```python
from build123d import *

# Parameters (mm, degrees)
EXTRUDE_366_DEPTH           = 3.75
EXTRUDE_366_TAPER           = 4.000000000000009
EXTRUDE_366_OTHER_WAY_DEPTH = 3.75
EXTRUDE_366_OTHER_WAY_TAPER = 4.000000000000009
EXTRUDE_746_DEPTH           = 3.75
EXTRUDE_746_TAPER           = 4.000000000000009
CUT_EXTRUDE_1239_DEPTH      = 10
SKETCH_4_R                  = 10
CUT_EXTRUDE_1_DEPTH         = 10
EXTRUDE_1783_DEPTH          = 7
FILLET_2_R                  = 2
FILLET_3_R                  = 2


with BuildPart() as part:
    # Эскиз1 → Extrude 366 (new body)
    with BuildSketch(Plane.XY):
        with BuildLine():
            ThreePointArc((-0.9374999999999997, 14.970674458754353), (-15.000000000000044, 1.84e-15), (-0.9374999999999997, -14.970674458754353))
            Line((-0.9374999999999997, -14.970674458754353), (78.75, -19.960899278339134))
            ThreePointArc((78.75, -19.960899278339134), (100, 0), (78.75, 19.960899278339134))
            Line((78.75, 19.960899278339134), (-0.9374999999999997, 14.970674458754353))
        make_face()
    extrude(amount=EXTRUDE_366_DEPTH, taper=EXTRUDE_366_TAPER)

    # Эскиз1 → Extrude 366 other way (add)
    with BuildSketch(Plane.XY):
        with BuildLine():
            ThreePointArc((-0.9374999999999997, 14.970674458754353), (-15.000000000000044, 1.84e-15), (-0.9374999999999997, -14.970674458754353))
            Line((-0.9374999999999997, -14.970674458754353), (78.75, -19.960899278339134))
            ThreePointArc((78.75, -19.960899278339134), (100, 0), (78.75, 19.960899278339134))
            Line((78.75, 19.960899278339134), (-0.9374999999999997, 14.970674458754353))
        make_face()
    extrude(amount=-EXTRUDE_366_OTHER_WAY_DEPTH, taper=EXTRUDE_366_OTHER_WAY_TAPER)

    # Эскиз2 → Extrude 746 (add)
    with BuildSketch(Plane.XY):
        with BuildLine():
            Line((-8.829475928589163, 70.3052843721409), (28.552506867722524, 0))
            Line((28.552506867722524, 0), (62.650318248221396, 1.896e-14))
            Line((62.650318248221396, 1.896e-14), (8.2903757255504, 80.59192903470749))
            ThreePointArc((8.2903757255504, 80.59192903470749), (-5.150380749100648, 83.57167300702106), (-8.829475928589163, 70.3052843721409))
        make_face()
    extrude(amount=EXTRUDE_746_DEPTH, taper=EXTRUDE_746_TAPER)

    # Эскиз3 → Cut-Extrude 1239 (cut)
    with BuildSketch(Plane.XY.offset(3.75)):
        with BuildLine():
            Line((3.464101615137748, 77.00000000000001), (23.464101615137906, 42.35898384862258))
            ThreePointArc((23.464101615137906, 42.35898384862258), (22.00000000000019, 36.89488223348481), (16.53589838486241, 38.358983848622536))
            Line((16.53589838486241, 38.358983848622536), (-3.464101615137746, 72.99999999999997))
            ThreePointArc((-3.464101615137746, 72.99999999999997), (-2.00000000000002, 78.46410161513775), (3.464101615137748, 77.00000000000001))
        make_face()
    extrude(amount=-CUT_EXTRUDE_1239_DEPTH, mode=Mode.SUBTRACT)

    # Эскиз4 → отверстие1 (cut)
    with BuildSketch(Plane.XY.offset(3.75)):
        Circle(SKETCH_4_R)
    extrude(amount=-CUT_EXTRUDE_1_DEPTH, mode=Mode.SUBTRACT)

    # Эскиз5 → Extrude 1783 (add)
    with BuildSketch(Plane.XY.offset(3.75)):
        Polygon((79.99999999999999, 13.856406460551018), (68, 6.928203230275526), (68, -6.9282032302754955), (80, -13.856406460551012), (92, -6.928203230275516), (92, 6.928203230275502), align=None)
    extrude(amount=EXTRUDE_1783_DEPTH)

    # Скругление2
    fillet_2_edges = [part.edges().sort_by_distance(p)[0] for p in [
        (99.73777445521183, -1.332e-14, -3.75),
        (99.73777445521183, -3.77e-15, 3.7499999999999996),
        (9.700092064405581, 15.374087104269854, 3.7499999999999987),
        (-14.737774455211877, -5.44e-15, 3.7499999999999996),
        (38.922639096549254, -17.204073984160544, 3.750000000000001),
        (38.922639096549226, 17.20407398416053, -3.75),
        (64.50880005583919, 18.806341534992715, 3.7499999999999996),
        (-14.737774455211884, -4.44e-15, -3.75),
        (38.92263909654925, -17.204073984160534, -3.75),
    ]]
    fillet(fillet_2_edges, radius=FILLET_2_R)

    # Скругление3
    fillet_3_edges = [part.edges().sort_by_distance(p)[0] for p in [
        (6.342464766178029, 42.32956867017836, 3.7500000000000004),
        (-5.0153246093207, 83.34690184461985, 3.7499999999999996),
        (29.766776124769358, 48.282920306520026, 3.7499999999999885),
    ]]
    fillet(fillet_3_edges, radius=FILLET_3_R)


solid = part.part
```
Here's how the part is built. I have some questions about the finished solid (model axes, mm). A direction names the side the tool comes from. Coordinates: 2 decimals unless noted, no trailing zeros. Use a Markdown table: item, result. Add a question column.
(1) I'm going to push flat-ended pins straight in: P1, Ø1, axis at y = -7.5, z = -2, coming from the -X side; P2, Ø2, axis at y = 3, z = 9, coming from the +X side; P3, Ø8, axis at x = 17, z = 0.5, coming from the +Y side; P4, Ø16, axis at x = 0, y = 0, coming from the +Z side. Where does each tip first touch, or does it pass through?
(2) We'd pull the mould along Y, two halves only. Please class faces 1 (the flat face through (92, 0, 7)), 2 (the cylindrical face through (28.759, 48.909, 3.198)), 3 (the flat face through (13.324, 59.922, 1.901)): +Y half, -Y half, draft (parallel to the pull), parting line (faces both ways), or undercut.
(3) For faces 4 (the cylindrical face through (63.8, 18.24, 3.23)), 5 (the flat face through (74.08, 10.44, 7.2)), 6 (the flat face through (39.468, -17.436, 0.932)), 7 (the flat face through (6.676, 55.437, 1.901)), which set-ups out of +Z, -Z, +X, -X, +Y, -Y let a thin tool reach every point of the face, with its end or its side?
(4) Please list where these lines run through material, in increasing order: line 1 (Y direction, x = -7, z = 1.75); line 2 (Y direction, x = 0, z = -0.5); line 3 (Y direction, x = 6, z = 3).
Outcome:
| question | item | result |
|---|---|---|
| 1 | P1 | stops at x = -13.11 |
| 1 | P2 | stops at x = 92 |
| 1 | P3 | stops at y = 73.57 |
| 1 | P4 | passes through |
| 2 | face 1 | draft |
| 2 | face 2 | +Y half |
| 2 | face 3 | undercut |
| 3 | face 4 | +Z, +Y |
| 3 | face 5 | +Z, -X, +Y |
| 3 | face 6 | +Z, -X, -Y |
| 3 | face 7 | +Z, -Z |
| 4 | line 1 | y = -13.13 to -7.14, 7.14 to 13.13, 67.13 to 81.97 |
| 4 | line 2 | y = -14.99 to -10, 10 to 14.99 |
| 4 | line 3 | y = -14.84 to -8, 8 to 14.84, 43.62 to 56.61, 72.61 to 82.28 |
